Could you check a few things on this model? Use its own coordinates, in mm. A direction names the side the tool comes from. Round coordinates to 2 decimals unless told otherwise and drop trailing zeros. Loops run counter-clockwise (first coordinate to the right, second up) from the corner with the lowest first, then second, coordinate; pieces in that order, holes last. Notation, with made-up numbers: (61, 77) -> (115, 77) arc R11 cw to (115, 91) -> close; hole circle Ø11 at (71.25, 58). An arc over 180 degrees is marked (long way). One line per item, written item: value.
Autodesk Inventor part; units mm, degrees
ref_plane "YZ Plane" through (0, 0, 0) normal (1, 0, 0) x (0, 1, 0)
ref_plane "XZ Plane" through (0, 0, 0) normal (0, 1, 0) x (-1, 0, 0)
ref_plane "XY Plane" through (0, 0, 0) normal (0, 0, 1) x (1, 0, 0)
sketch "Boceto1" plane through (0, 0, 0) normal (0, 1, 0) x (-1, 0, 0)
  line L0 (112.646, 23.1115) -> (33.646, 23.1115)
  circle A0 centre (89.8586, 65.5785) radius 1.5
  circle A1 centre (89.8586, 65.5785) radius 1.5
  circle A2 centre (103.0678, 65.5785) radius 1.5
  line L1 (103.0678, 65.5785) -> (103.0678, 30.5785)
  circle A3 centre (103.0678, 30.5785) radius 1.5
  line L2 (103.0678, 30.5785) -> (99.0678, 30.5785)
  line L3 (99.0678, 30.5785) -> (99.0678, 25.5785)
  line L4 (99.0678, 25.5785) -> (107.0678, 25.5785)
  line L5 (107.0678, 25.5785) -> (107.0678, 75.5785)
  line L6 (107.0678, 75.5785) -> (99.0678, 75.5785)
  line L7 (99.0678, 75.5785) -> (99.0678, 25.5785)
  point P0 (0, 0)
  dimension "d0" = 35
  dimension "d1" = 3
  dimension "d2" = 4
  dimension "d3" = 5
  dimension "d4" = 8
  dimension "d5" = 50
extrude "Extrusión1" add sketch "Boceto1" along normal blind 2 contours L7 L6 L5 L4 L3
thicken "Engrosado1" operation add thickness 2.467 both sides no extend neighbours yes toward (0, 0, -1) faces at (-101.7345, 0.6667, 25.5785)
sketch "Boceto2" plane through (0, 2, 0) normal (0, 1, 0) x (1, 0, 0)
  line L0 (-99.0678, -23.1115) -> (-107.0678, -23.1115)
  line L1 (-99.0678, -75.5785) -> (-99.0678, -23.1115)
  line L2 (-107.0678, -23.1115) -> (-99.0678, -23.1115)
  line L3 (-99.0678, -23.1115) -> (-99.0678, -26.1115)
  line L4 (-99.0678, -26.1115) -> (-107.0678, -26.1115)
  line L5 (-107.0678, -26.1115) -> (-107.0678, -23.1115)
  point P0 (0, 0)
  dimension "d10" = 3
extrude "Extrusión2" add sketch "Boceto2" along normal blind 91
properties part number "soporte3pantalla"
Item 1: If we mould it in two halves opening along Z, with no side actions, what happens to faces 1 (the face through (-103, 47, 26.112)), 2 (the face through (-103, 0, 50)), 3 (the face through (-101.57, 0.99, 30.51))? For each: released by +Z, released by -Z, zero draft, split by the parting line, or undercut.
Output:
face 1: released by +Z
face 2: zero draft
face 3: undercut
Item 2: If we section it at B-B on z = 58.5: List the corners of the cut face in (x, y) for me, plus the area to 3 significant figures.
Output:
outline: (-107.07, 0) -> (-99.07, 0) -> (-99.07, 2) -> (-107.07, 2) -> close
area: 16.0 mm²
Item 3: Will this pin go through, and if not, where does the flat tip stop? pin 1 Ø2 at (x, y) = (-103.5, 63.5) entering from +Z.
Output:
pin 1: stops at z = 26.11
Item 4: I need wall thicknesses on line 1 (Z direction, x = -103.25, y = 28.5); line 2 (Y direction, x = -100.75, z = 54.5). Which ranges of each line are inside material? Lowest first, please. Write a range as from..to.
Output:
line 1: z = 23.11..26.11
line 2: y = 0..2
Item 5: If we section it at C-C on y = 67: List the corners of the cut face in (x, z) for me.
Output:
outline: (-107.07, 23.11) -> (-99.07, 23.11) -> (-99.07, 26.11) -> (-107.07, 26.11) -> close
Item 6: If we section it at A-A on x = -102.5: List the corners of the cut face in (y, z) for me.
Output:
outline: (0, 23.11) -> (93, 23.11) -> (93, 26.11) -> (2, 26.11) -> (2, 29.19) -> (0, 29.19) -> close; (0, 31.97) -> (2, 31.97) -> (2, 64.19) -> (0, 64.19) -> close; (0, 66.97) -> (2, 66.97) -> (2, 75.58) -> (0, 75.58) -> close
Item 7: For faces 4 (the face through (-103, 93, 25)), 5 (the face through (-103, 2, 51)), which set-ups out of +Z, -Z, +X, -X, +Y, -Y let a thin tool reach every point of the face, with its end or its side?
Output:
face 4: +Z, -Z, +X, -X, +Y
face 5: +Z, +X, -X, +Y
